For this review, take the finished solid that the model builds, in its own axes (mm). A direction names the side the tool comes from. Round coordinates to 2 decimals unless told otherwise and drop trailing zeros. Order: outer loops, then holes, each group sorted by start corner. A loop starts at its lowest first (then second) coordinate and runs counter-clockwise, first axis right, second up. Notation, with made-up numbers: (20, -32.75) -> (56, -32.75) arc R25 ccw to (56, -0.75) -> close; hole circle Ø5 at (26, 47). An arc over 180 degrees is marked (long way). Answer in a Markdown table with one row per item.
Autodesk Inventor part; units mm, degrees
ref_plane "YZ Plane" through (0, 0, 0) normal (1, 0, 0) x (0, 1, 0)
ref_plane "XZ Plane" through (0, 0, 0) normal (0, 1, 0) x (-1, 0, 0)
ref_plane "XY Plane" through (0, 0, 0) normal (0, 0, 1) x (1, 0, 0)
sketch "Эскиз1" plane through (0, 0, 0) normal (0, 0, 1) x (1, 0, 0)
  line L0 (-30, 41.5) -> (28, 41.5)
  line L1 (30, 39.5) -> (30, -39.5)
  line L2 (28, -41.5) -> (-30, -41.5)
  line L3 (-30, -41.5) -> (-30, 41.5)
  line L4 (-30, 41.5) -> (30, -41.5) construction
  line L5 (30, 41.5) -> (-30, -41.5) construction
  line L6 (-30, -41.5) -> (-42.5, -41.5)
  line L7 (-46.5, -37.5) -> (-46.5, 37.5)
  line L8 (-42.5, 41.5) -> (-30, 41.5)
  line L9 (-30, 41.5) -> (-30, -41.5)
  line L10 (-42.5, -41.5) -> (-46.5, -37.5)
  line L11 (-46.5, 37.5) -> (-42.5, 41.5)
  line L12 (28, 41.5) -> (30, 39.5)
  line L13 (28, -41.5) -> (30, -39.5)
  line L14 (0, 0) -> (-23.984, 0) construction
  line L15 (-23.984, 0) -> (-23.984, 15.7) construction
  line L16 (-23.984, 15.7) -> (0, 15.7) construction
  line L17 (0, 15.7) -> (0, 0) construction
  circle A0 centre (-23.984, 15.7) radius 1.6
  circle A1 centre (-23.984, -15.7) radius 1.6
  circle A2 centre (23.984, 15.7) radius 1.6
  circle A3 centre (23.984, -15.7) radius 1.6
  line L18 (-46.5, -41.5) -> (-25.168, -41.5)
  line L19 (-25.168, -41.5) -> (-25.168, -21.7)
  line L20 (-29.168, -17.7) -> (-46.5, -17.7)
  line L21 (-46.5, -17.7) -> (-46.5, -41.5)
  arc A4 (-25.168, -21.7) -> (-29.168, -17.7) centre (-29.168, -21.7) ccw
  line L22 (-25.168, 41.5) -> (-25.168, 21.7)
  line L23 (-29.168, 17.7) -> (-46.5, 17.7)
  arc A5 (-29.168, 17.7) -> (-25.168, 21.7) centre (-29.168, 21.7) ccw
  point P0 (-46.5, 41.5)
  point P1 (-25.168, -17.7)
  point P2 (-25.168, 41.5)
  point P3 (-46.5, -17.7)
  point P4 (-25.168, -41.5)
  dimension "d0" = 60
  dimension "d1" = 83
  dimension "d2" = 16.5
  dimension "d3" = 83
  dimension "d6" = 4
  dimension "d7" = 4
  dimension "d8" = 4
  dimension "d9" = 4
  dimension "d10" = 2
  dimension "d11" = 2
  dimension "d12" = 2
  dimension "d13" = 2
  dimension "d14" = 23.984
  dimension "d15" = 15.7
  dimension "d16" = 3.2
  dimension "d17" = 21.332
  dimension "d18" = 23.8
  dimension "d19" = 4
extrude "Выдавливание1" add sketch "Эскиз1" along normal blind 1.5 contours L0 L12 L1 L13 L2 L19 A4 L20 L3 L23 A5 L22 | L3 L20 L7 L23 | A0 | A1 | A2 | A3
chamfer "Фаска1" distance 2 angle 45 4 edges at (-46.5, -17.7, 0.75) (-46.5, 17.7, 0.75) (-25.168, -41.5, 0.75) (-25.168, 41.5, 0.75)
sketch "Эскиз2" plane through (0, 0, 0) normal (0, 0, -1) x (-1, 0, 0)
  arc A0 (43.584, 19.7) -> (47.584, 23.7) centre (43.584, 23.7) ccw
  arc A1 (27.668, 34.3) -> (26.418, 35.8612) centre (26.068, 34.3) ccw
  line L0 (27.668, 34.3) -> (27.668, 31.0225)
  arc A2 (26.418, 29.4612) -> (27.668, 31.0225) centre (26.068, 31.0225) ccw
  arc A3 (26.418, 29.4612) -> (25.168, 27.9) centre (26.768, 27.9) ccw
  line L1 (25.168, 27.9) -> (25.168, 23.7)
  arc A4 (25.168, 23.7) -> (29.168, 19.7) centre (29.168, 23.7) ccw
  line L2 (29.168, 19.7) -> (43.584, 19.7)
  arc A5 (43.584, 19.7) -> (47.584, 23.7) centre (43.584, 23.7) ccw
  line L3 (47.584, 23.7) -> (47.584, 39.2)
  line L4 (47.584, 39.2) -> (25.168, 39.2)
  line L5 (25.168, 39.2) -> (25.168, 37.4225)
  arc A6 (25.168, 37.4225) -> (26.418, 35.8612) centre (26.768, 37.4225) ccw
  line L6 (52.084, -4) -> (58.0913, -4)
  line L7 (58.0913, -4) -> (58.0913, -38.5)
  line L8 (58.0913, -38.5) -> (69.3773, -38.5)
  line L9 (69.3773, -38.5) -> (69.3773, 32.5)
  line L10 (69.3773, 32.5) -> (58.0913, 32.5)
  line L11 (58.0913, 32.5) -> (58.0913, 24)
  line L12 (58.0913, 24) -> (52.084, 24)
  line L13 (52.084, 24) -> (52.084, 13.5)
  line L14 (52.084, 13.5) -> (34.584, 13.5)
  arc A7 (34.584, 13.5) -> (34.584, 1.5) centre (34.584, 7.5) ccw
  line L15 (34.584, 1.5) -> (47.084, 1.5)
  line L16 (47.084, 1.5) -> (47.084, -3.7639)
  spline S0 degree 3 poles (48.084, -6) (47.8036, -5.6035) (47.4716, -5.1246) (47.1717, -4.4032) (47.084, -4.0595) (47.084, -3.7639) knots 0.566831 0.566831 0.566831 0.566831 0.71252 0.71252 0.801197 0.801197 0.801197 0.801197
  line L17 (51.084, -6) -> (48.084, -6)
  spline S1 degree 3 poles (52.084, -3.7639) (52.084, -4.0595) (51.9963, -4.4032) (51.6964, -5.1246) (51.3644, -5.6035) (51.084, -6) knots 0 0 0 0 0.088677 0.088677 0.234365 0.234365 0.234365 0.234365
  line L18 (52.084, -3.7639) -> (52.084, -4)
  line L19 (74.484, -42.6) -> (-79.316, -42.6)
  line L20 (-79.316, -42.6) -> (-79.316, 42.6)
  line L21 (6.584, 42.6) -> (74.484, 42.6)
  line L22 (74.484, 42.6) -> (74.484, -42.6)
  circle A8 centre (23.684, -32.7) radius 1.6
  circle A9 centre (23.684, 32.7) radius 1.6
  line L23 (20.484, 41.2) -> (6.584, 41.2)
  line L24 (-25.316, 41.2) -> (-25.316, -41.2)
  line L25 (-25.316, -41.2) -> (20.484, -41.2)
  line L26 (20.484, -41.2) -> (20.484, 41.2)
  circle A10 centre (-28.516, -32.7) radius 1.6
  circle A11 centre (-28.516, 32.7) radius 1.6
  arc A12 (-32.5, 31.0225) -> (-31.25, 29.4612) centre (-30.9, 31.0225) ccw
  line L27 (-32.5, 31.0225) -> (-32.5, 34.3775)
  arc A13 (-31.25, 35.9388) -> (-32.5, 34.3775) centre (-30.9, 34.3775) ccw
  arc A14 (-31.25, 35.9388) -> (-30, 37.5) centre (-31.6, 37.5) ccw
  line L28 (-30, 37.5) -> (-30, 39.2)
  line L29 (-30, 39.2) -> (-52.416, 39.2)
  line L30 (-52.416, 39.2) -> (-52.416, 23.7)
  arc A15 (-52.416, 23.7) -> (-48.416, 19.7) centre (-48.416, 23.7) ccw
  line L31 (-48.416, 19.7) -> (-34, 19.7)
  arc A16 (-34, 19.7) -> (-30, 23.7) centre (-34, 23.7) ccw
  line L32 (-30, 23.7) -> (-30, 27.9)
  arc A17 (-30, 27.9) -> (-31.25, 29.4612) centre (-31.6, 27.9) ccw
  arc A18 (-32.5, -34.3) -> (-31.25, -35.8612) centre (-30.9, -34.3) ccw
  line L33 (-32.5, -34.3) -> (-32.5, -31.0225)
  arc A19 (-31.25, -29.4612) -> (-32.5, -31.0225) centre (-30.9, -31.0225) ccw
  arc A20 (-31.25, -29.4612) -> (-30, -27.9) centre (-31.6, -27.9) ccw
  line L34 (-30, -27.9) -> (-30, -23.7)
  arc A21 (-30, -23.7) -> (-34, -19.7) centre (-34, -23.7) ccw
  line L35 (-34, -19.7) -> (-48.416, -19.7)
  arc A22 (-48.416, -19.7) -> (-52.416, -23.7) centre (-48.416, -23.7) ccw
  line L36 (-52.416, -23.7) -> (-52.416, -39.2)
  line L37 (-52.416, -39.2) -> (-30, -39.2)
  line L38 (-30, -39.2) -> (-30, -37.4225)
  arc A23 (-30, -37.4225) -> (-31.25, -35.8612) centre (-31.6, -37.4225) ccw
  arc A24 (26.418, -35.9388) -> (27.668, -34.3775) centre (26.068, -34.3775) ccw
  arc A25 (26.418, -35.9388) -> (25.168, -37.5) centre (26.768, -37.5) ccw
  line L39 (25.168, -37.5) -> (25.168, -39.2)
  line L40 (25.168, -39.2) -> (47.584, -39.2)
  line L41 (47.584, -39.2) -> (47.584, -23.7)
  arc A26 (47.584, -23.7) -> (43.584, -19.7) centre (43.584, -23.7) ccw
  line L42 (43.584, -19.7) -> (29.168, -19.7)
  arc A27 (29.168, -19.7) -> (25.168, -21.7) centre (29.168, -23.7) ccw
  line L43 (25.168, -21.7) -> (25.168, -27.9)
  arc A28 (25.168, -27.9) -> (26.418, -29.4612) centre (26.768, -27.9) ccw
  arc A29 (27.668, -31.0225) -> (26.418, -29.4612) centre (26.068, -31.0225) ccw
  line L44 (27.668, -31.0225) -> (27.668, -34.3775)
  line L45 (25.168, -39.2) -> (25.168, 39.2)
  line L46 (25.168, -21.7) -> (25.168, -39.5)
  line L47 (-30, 39.2) -> (-30, -39.2)
  line L48 (-11.416, 42.6) -> (-11.416, 41.2)
  line L49 (-11.416, 41.2) -> (-25.316, 41.2)
  line L50 (6.584, 41.2) -> (6.584, 42.6)
  line L51 (-79.316, 42.6) -> (-11.416, 42.6)
  point P0 (0, 0)
  point P1 (-30, -37.4225)
  point P2 (-30, -27.9)
  point P3 (-30, 27.9)
  point P4 (-30, 37.5)
  point P5 (25.168, 37.4225)
  point P6 (25.168, 27.9)
  point P7 (25.168, -37.5)
  point P8 (25.168, -27.9)
extrude "Выдавливание2" add sketch "Эскиз2" against normal blind 1.5 contours L45 A9 A6 A1 L0 A2 A3 | L45 A9 | A28 A29 L44 A24 A25 L45 A8 | A8 L45 | L47 A10 | A10 L47 A23 A18 L33 A19 A20 | A17 A12 L27 A13 A14 L47 A11 | A11 L47 picked at (25.1894, 32.5653) picked at (25.1894, -32.5653) picked at (-30.0289, -32.5985) picked at (-30.0289, 32.8015)
sketch "Эскиз3" plane through (0, 0, 0) normal (0, 0, -1) x (-1, 0, 0)
  arc A0 (27.668, 34.3) -> (26.418, 35.8612) centre (26.068, 34.3) ccw
  line L0 (27.668, 34.3) -> (27.668, 31.0225)
  arc A1 (26.418, 29.4612) -> (27.668, 31.0225) centre (26.068, 31.0225) ccw
  arc A2 (26.418, 29.4612) -> (25.168, 27.9) centre (26.768, 27.9) ccw
  line L1 (25.168, 27.9) -> (25.168, 23.7)
  arc A3 (25.168, 23.7) -> (29.168, 19.7) centre (29.168, 23.7) ccw
  line L2 (29.168, 19.7) -> (43.584, 19.7)
  arc A4 (43.584, 19.7) -> (47.584, 23.7) centre (43.584, 23.7) ccw
  line L3 (47.584, 23.7) -> (47.584, 39.2)
  line L4 (47.584, 39.2) -> (25.168, 39.2)
  line L5 (25.168, 39.2) -> (25.168, 37.4225)
  arc A5 (25.168, 37.4225) -> (26.418, 35.8612) centre (26.768, 37.4225) ccw
  line L6 (52.084, -4) -> (58.0913, -4)
  line L7 (58.0913, -4) -> (58.0913, -38.5)
  line L8 (58.0913, -38.5) -> (69.3773, -38.5)
  line L9 (69.3773, -38.5) -> (69.3773, 32.5)
  line L10 (69.3773, 32.5) -> (58.0913, 32.5)
  line L11 (58.0913, 32.5) -> (58.0913, 24)
  line L12 (58.0913, 24) -> (52.084, 24)
  line L13 (52.084, 24) -> (52.084, 13.5)
  line L14 (52.084, 13.5) -> (34.584, 13.5)
  arc A6 (34.584, 13.5) -> (34.584, 1.5) centre (34.584, 7.5) ccw
  line L15 (34.584, 1.5) -> (47.084, 1.5)
  line L16 (47.084, 1.5) -> (47.084, -3.7639)
  spline S0 degree 3 poles (48.084, -6) (47.8036, -5.6035) (47.4716, -5.1246) (47.1717, -4.4032) (47.084, -4.0595) (47.084, -3.7639) knots 0.566831 0.566831 0.566831 0.566831 0.71252 0.71252 0.801197 0.801197 0.801197 0.801197
  line L17 (51.084, -6) -> (48.084, -6)
  spline S1 degree 3 poles (52.084, -3.7639) (52.084, -4.0595) (51.9963, -4.4032) (51.6964, -5.1246) (51.3644, -5.6035) (51.084, -6) knots 0 0 0 0 0.088677 0.088677 0.234365 0.234365 0.234365 0.234365
  line L18 (52.084, -3.7639) -> (52.084, -4)
  line L19 (74.484, -42.6) -> (-79.316, -42.6)
  line L20 (-79.316, -42.6) -> (-79.316, 42.6)
  line L21 (6.584, 42.6) -> (74.484, 42.6)
  line L22 (74.484, 42.6) -> (74.484, -42.6)
  circle A7 centre (23.684, -32.7) radius 1.6
  circle A8 centre (23.684, 32.7) radius 1.6
  line L23 (20.484, 41.2) -> (6.584, 41.2)
  line L24 (-25.316, 41.2) -> (-25.316, -41.2)
  line L25 (-25.316, -41.2) -> (20.484, -41.2)
  line L26 (20.484, -41.2) -> (20.484, 41.2)
  circle A9 centre (-28.516, -32.7) radius 1.6
  circle A10 centre (-28.516, 32.7) radius 1.6
  arc A11 (-32.5, 31.0225) -> (-31.25, 29.4612) centre (-30.9, 31.0225) ccw
  line L27 (-32.5, 31.0225) -> (-32.5, 34.3775)
  arc A12 (-31.25, 35.9388) -> (-32.5, 34.3775) centre (-30.9, 34.3775) ccw
  arc A13 (-31.25, 35.9388) -> (-30, 37.5) centre (-31.6, 37.5) ccw
  line L28 (-30, 37.5) -> (-30, 39.2)
  line L29 (-30, 39.2) -> (-52.416, 39.2)
  line L30 (-52.416, 39.2) -> (-52.416, 23.7)
  arc A14 (-52.416, 23.7) -> (-48.416, 19.7) centre (-48.416, 23.7) ccw
  line L31 (-48.416, 19.7) -> (-34, 19.7)
  arc A15 (-34, 19.7) -> (-30, 23.7) centre (-34, 23.7) ccw
  line L32 (-30, 23.7) -> (-30, 27.9)
  arc A16 (-30, 27.9) -> (-31.25, 29.4612) centre (-31.6, 27.9) ccw
  arc A17 (-32.5, -34.3) -> (-31.25, -35.8612) centre (-30.9, -34.3) ccw
  line L33 (-32.5, -34.3) -> (-32.5, -31.0225)
  arc A18 (-31.25, -29.4612) -> (-32.5, -31.0225) centre (-30.9, -31.0225) ccw
  arc A19 (-31.25, -29.4612) -> (-30, -27.9) centre (-31.6, -27.9) ccw
  line L34 (-30, -27.9) -> (-30, -23.7)
  arc A20 (-30, -23.7) -> (-34, -19.7) centre (-34, -23.7) ccw
  line L35 (-34, -19.7) -> (-48.416, -19.7)
  arc A21 (-48.416, -19.7) -> (-52.416, -23.7) centre (-48.416, -23.7) ccw
  line L36 (-52.416, -23.7) -> (-52.416, -39.2)
  line L37 (-52.416, -39.2) -> (-30, -39.2)
  line L38 (-30, -39.2) -> (-30, -37.4225)
  arc A22 (-30, -37.4225) -> (-31.25, -35.8612) centre (-31.6, -37.4225) ccw
  arc A23 (26.418, -35.9388) -> (27.668, -34.3775) centre (26.068, -34.3775) ccw
  arc A24 (26.418, -35.9388) -> (25.168, -37.5) centre (26.768, -37.5) ccw
  line L39 (25.168, -37.5) -> (25.168, -39.2)
  line L40 (25.168, -39.2) -> (47.584, -39.2)
  line L41 (47.584, -39.2) -> (47.584, -23.7)
  arc A25 (47.584, -23.7) -> (43.584, -19.7) centre (43.584, -23.7) ccw
  line L42 (43.584, -19.7) -> (29.168, -19.7)
  arc A26 (29.168, -19.7) -> (25.168, -23.7) centre (29.168, -23.7) ccw
  line L43 (25.168, -23.7) -> (25.168, -27.9)
  arc A27 (25.168, -27.9) -> (26.418, -29.4612) centre (26.768, -27.9) ccw
  arc A28 (27.668, -31.0225) -> (26.418, -29.4612) centre (26.068, -31.0225) ccw
  line L44 (27.668, -31.0225) -> (27.668, -34.3775)
  line L45 (25.168, -39.5) -> (23.168, -41.5)
  line L46 (23.168, -41.5) -> (25.168, -41.5) construction
  line L47 (25.168, -41.5) -> (25.168, -39.5) construction
  line L48 (25.168, -39.5) -> (23.168, -39.5) construction
  line L49 (23.168, -39.5) -> (23.168, -41.5) construction
  line L50 (25.168, -41.5) -> (-15.416, -41.5) construction
  line L51 (-15.416, -41.5) -> (-15.416, -24.5) construction
  line L52 (-15.416, -24.5) -> (25.168, -24.5) construction
  line L53 (25.168, -24.5) -> (25.168, -41.5) construction
  circle A29 centre (-15.416, -24.5) radius 1.5
  line L54 (-25.316, 0) -> (20.484, 0) construction
  circle A30 centre (-15.416, 24.5) radius 1.5
  circle A31 centre (23.684, -32.7) radius 1.35
  circle A32 centre (-28.516, -32.7) radius 1.35
  circle A33 centre (-28.516, 32.7) radius 1.35
  circle A34 centre (23.684, 32.7) radius 1.35
  line L55 (-11.416, 42.6) -> (-11.416, 41.2)
  line L56 (-11.416, 41.2) -> (-25.316, 41.2)
  line L57 (6.584, 41.2) -> (6.584, 42.6)
  line L58 (-79.316, 42.6) -> (-11.416, 42.6)
  point P0 (0, 0)
  dimension "d25" = 40.584
  dimension "d26" = 17
  dimension "d27" = 3
  dimension "d28" = 2.7
  dimension "d29" = 2.7
  dimension "d30" = 2.7
  dimension "d31" = 2.7
extrude "Выдавливание3" cut sketch "Эскиз3" against normal blind 1.5 contours A29 | A30 | A31 | A32 | A33 | A34
equation "\"d7\" = d6"
equation "\"d11\" = d10"
properties part number "power_board"
Q1. Clearance check with a flat-ended pin moving along its axis: pin 1 Ø0.8 at (y, z) = (26.5, 1) entering from -X. State where the tip first meets the part, or that it passes through.
Answer key:
| item | result |
|---|---|
| pin 1 | stops at x = -25.17 |
Q2. The part is to be moulded in two halves that separate along X. For faces 3 (the face through (1, 1, 1.5)), 4 (the face through (29, 40.5, 0.7)), 5 (the face through (-23.51, -31.36, 0.74)), say which applies: +X half, -X half, draft (parallel to the pull), parting line (faces both ways), or undercut.
Answer key:
| item | result |
|---|---|
| face 3 | draft |
| face 4 | +X half |
| face 5 | undercut |
Q3. Take a section at B-B, the plane z = 1.1. Give the number of separate pieces and of enclosed holes in the cut face, then the cut area to 3 significant figures.
Answer key:
| item | result |
|---|---|
| separate pieces | 1 |
| enclosed holes | 6 |
| area | 5,360 mm^2 |
Q4. Tool access review of faces 1 (the face through (1, 1, 0)), 2 (the face through (-26.31, 18.9, 0.74)): name each direction out of +Z, -Z, +X, -X, +Y, -Y from which nothing blocks a thin tool from reaching the whole face with its end or side.
Answer key:
| item | result |
|---|---|
| face 1 | -Z, +X, -X, +Y, -Y |
| face 2 | +Z, -Z, -X |
Q5. Take a section at A-A, the plane y = 24.5. Write out the cut boundary in (x, z).
Answer key:
| item | result |
|---|---|
| outline | (-25.17, 0) -> (13.92, 0) -> (13.92, 1.5) -> (-25.17, 1.5) -> close; (16.92, 0) -> (30, 0) -> (30, 1.5) -> (16.92, 1.5) -> close |
Q6. To check wall thickness, follow probe 1 along Y at (x, z) = (-27, 0.8); probe 2 along X at (y, z) = (-4, 0.65); probe 3 along Y at (x, z) = (-38, 0.2). State the ranges of each line that lie inside material, in increasing order.
Answer key:
| item | result |
|---|---|
| probe 1 | y = -35.68 to -29.72, -18.34 to 18.34, 29.72 to 35.6 |
| probe 2 | x = -46.5 to 30 |
| probe 3 | y = -17.7 to 17.7 |
Q7. Take a section at C-C, the plane y = 4.5. Write out the cut boundary in (x, z), then the cut area to 3 significant figures.
Answer key:
| item | result |
|---|---|
| outline | (-46.5, 0) -> (30, 0) -> (30, 1.5) -> (-46.5, 1.5) -> close |
| area | 115 mm^2 |
